from build123d import *

# Parameters (mm, degrees)
AUFSATZ_LINEAR_AUSTRAGEN1_DEPTH = 5


with BuildPart() as part:
    # Skizze1 → Aufsatz-Linear austragen1 (new body)
    with BuildSketch(Plane.XY):
        with BuildLine():
            Line((-61.378328771, 63.819239112), (-56.378328771, 63.819239112))
            Line((-56.378328771, 63.819239112), (-56.378328771, 6.977133849))
            Line((-56.378328771, 6.977133849), (-61.378328771, 6.977133849))
            Line((-61.378328771, 6.977133849), (-61.378328771, -9.921658625))
            Line((-61.378328771, -9.921658625), (-43.939454059, -9.921658625))
            Line((-43.939454059, -9.921658625), (-43.939454059, -4.921658625))
            Line((-43.939454059, -4.921658625), (16.060545941, -4.921658625))
            Line((16.060545941, -4.921658625), (16.060545941, -9.921658625))
            Line((16.060545941, -9.921658625), (33.621671229, -9.921658625))
            Line((33.621671229, -9.921658625), (33.621671229, 6.977133849))
            Line((33.621671229, 6.977133849), (28.621671229, 6.977133849))
            Line((28.621671229, 6.977133849), (28.621671229, 63.819239112))
            Line((28.621671229, 63.819239112), (33.621671229, 63.819239112))
            Line((33.621671229, 63.819239112), (33.621671229, 80.078341375))
            Line((33.621671229, 80.078341375), (26.121671229, 80.078341375))
            ThreePointArc((26.121671229, 80.078341375), (22.586137323, 78.613875281), (21.121671229, 75.078341375))
            Line((21.121671229, 75.078341375), (21.121671229, 35.078341375))
            ThreePointArc((21.121671229, 35.078341375), (-13.878328771, 23.078341375), (-48.878328771, 35.078341375))
            Line((-48.878328771, 35.078341375), (-48.878328771, 75.078341375))
            ThreePointArc((-48.878328771, 75.078341375), (-50.342794866, 78.613875281), (-53.878328771, 80.078341375))
            Line((-53.878328771, 80.078341375), (-61.378328771, 80.078341375))
            Line((-61.378328771, 80.078341375), (-61.378328771, 63.819239112))
        make_face()
    extrude(amount=AUFSATZ_LINEAR_AUSTRAGEN1_DEPTH)


solid = part.part
Model file for the job. Use its own axes, mm. A direction names the side the tool comes from. Round coordinates to 2 decimals unless told otherwise and drop trailing zeros. Loops run counter-clockwise (first coordinate to the right, second up) from the corner with the lowest first, then second, coordinate; pieces in that order, holes last.
1. Band-saw the part on C-C, the plane y = 25. List the corners of the cut face in (x, z).
Check values:
outline: (-56.38, 0) - (-28.56, 0) - (-28.56, 5) - (-56.38, 5) - close; (0.8, 0) - (28.62, 0) - (28.62, 5) - (0.8, 5) - close
2. Wall check: probe 1 along X at (y, z) = (56.5, 0.35); probe 2 along X at (y, z) = (22, 3.75); probe 3 along Y at (x, z) = (-12.5, 4.1) (3 decimals). Give the ranges that are in metal, low to high.
Check values:
probe 1: x = -56.38 to -48.88, 21.12 to 28.62
probe 2: x = -56.38 to 28.62
probe 3: y = -4.922 to 23.095
3. Band-saw the part on B-B, the plane z = 3.25. List the corners of the cut face in (x, y), and give its area (3 significant figures).
Check values:
outline: (-61.38, -9.92) - (-43.94, -9.92) - (-43.94, -4.92) - (16.06, -4.92) - (16.06, -9.92) - (33.62, -9.92) - (33.62, 6.98) - (28.62, 6.98) - (28.62, 63.82) - (33.62, 63.82) - (33.62, 80.08) - (26.12, 80.08) arc R5 ccw to (21.12, 75.08) - (21.12, 35.08) arc R57.04 cw to (-48.88, 35.08) - (-48.88, 75.08) arc R5 ccw to (-53.88, 80.08) - (-61.38, 80.08) - (-61.38, 63.82) - (-56.38, 63.82) - (-56.38, 6.98) - (-61.38, 6.98) - close
area: 3,950 mm2
4. Mould opens along Y. For faces 6 (the flat face through (28.622, 35, 2)), 7 (the flat face through (-4, 16, 5)), 8 (the flat face through (25, -9.922, 2)) say: +Y half, -Y half, draft (parallel to the pull), parting line (faces both ways), or undercut.
Check values:
face 6: undercut
face 7: draft
face 8: -Y half
5. Tool access for faces 1 (the flat face through (33.622, -2, 2)), 2 (the flat face through (-14, -4.922, 2)), 3 (the cylindrical face through (22.625, 78.653, 2.465)), 4 (the flat face through (-59, 6.977, 2)), 5 (the flat face through (31, 6.977, 2)): list every direction of +Z, -Z, +X, -X, +Y, -Y with a clear straight run to the whole face (end or side of a thin tool).
Check values:
face 1: +Z, -Z, +X, +Y, -Y
face 2: +Z, -Z, -Y
face 3: +Z, -Z, +Y
face 4: +Z, -Z, -X
face 5: +Z, -Z, +X
6. Band-saw the part on D-D, the plane y = 10. List the corners of the cut face in (x, z), and give its area (3 significant figures).
Check values:
outline: (-56.38, 0) - (28.62, 0) - (28.62, 5) - (-56.38, 5) - close
area: 425 mm2
7. Drop flat-ended pins along their axis: P1, Ø4, axis at x = 17.5, y = 48, coming from the +Z side; P2, Ø1.5, axis at y = 51.5, z = 2.5, coming from the -X side; P3, Ø2.5, axis at x = -0.5, z = 2.5, coming from the -Y side; P4, Ø2.5, axis at y = 51.5, z = 2.5, coming from the +X side. Give the stop position or say it passes through.
Check values:
P1: passes through
P2: stops at x = -56.38
P3: stops at y = -4.92
P4: stops at x = 28.62
8. Band-saw the part on A-A, the plane y = 59.5. List the corners of the cut face in (x, z), and give its area (3 significant figures).
Check values:
outline: (-56.38, 0) - (-48.88, 0) - (-48.88, 5) - (-56.38, 5) - close; (21.12, 0) - (28.62, 0) - (28.62, 5) - (21.12, 5) - close
area: 75.0 mm2
